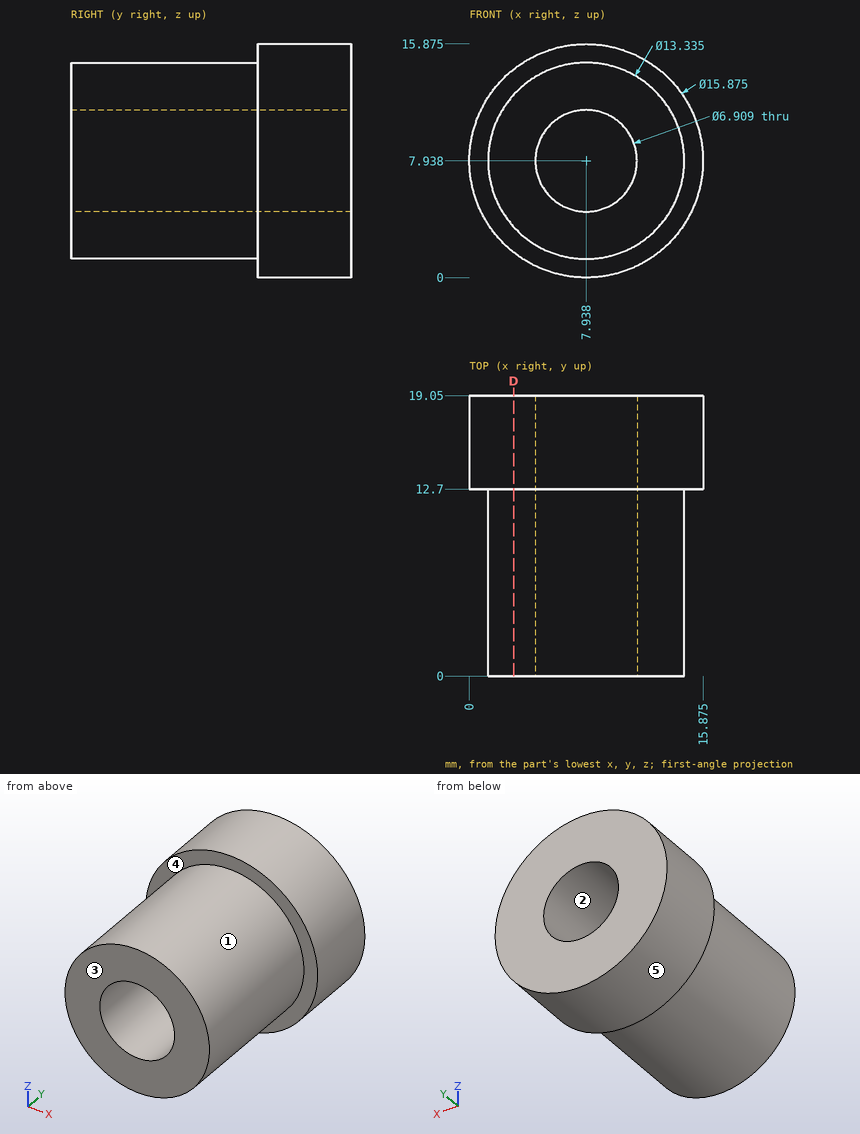
Design review of the part shown in the three views and the two pictorial views. Dimensions are in mm from the part's minimum x, y and z. A direction names the side the tool comes from. Give positions to 0.01 mm unless a question says otherwise; leave off trailing zeros. Write each loop counter-clockwise with the first axis right and the second up, starting at its lowest first coordinate (ties: lowest second). Pieces come first, ordered by that corner, then holes. Notation, with made-up numbers: M 76,33 L 103,33 A22 cw 103,48 Z; hole C 9,85 d4. An arc over 180 degrees is marked long. Answer in a Markdown table with one row per item.
Item 1: For P1, Ø3, axis at y = 15.5, z = 13, coming from the +X side; P2, Ø5, axis at x = 10.5, y = 10.5, coming from the -Z side; P3, Ø8, axis at x = 10.5, y = 10.5, coming from the -Z side; P4, Ø8, axis at y = 8, z = 11.5, coming from the +X side (1 decimal), all flat-tipped, find the tip position at first contact; note any pin that passes through.
Check sheet entries:
| item | result |
|---|---|
| P1 | x = 15.03 |
| P2 | z = 0.12 |
| P3 | z = 0 |
| P4 | x = 14.6 |
Item 2: Tool access review of the marked faces 4 and 5: name each direction out of +Z, -Z, +X, -X, +Y, -Y from which nothing blocks a thin tool from reaching the whole face with its end or side.
Check sheet entries:
| item | result |
|---|---|
| face 4 | -Y |
| face 5 | +Y, -Y |
Item 3: For line 1 along Z through (x, y) = (8, 8) (1 decimal); line 2 along Y through (x, z) = (4.25, 1.5), list the stretches that pass through material, from the lowest coordinate up.
Check sheet entries:
| item | result |
|---|---|
| line 1 | 1.3 to 4.5, 11.4 to 14.6 |
| line 2 | 12.7 to 19.05 |
Item 4: Draft analysis for pull direction X (two halves, no side actions). For the marked faces 1, 2 and 3, state which applies: +X half, -X half, draft (parallel to the pull), parting line (faces both ways), or undercut.
Check sheet entries:
| item | result |
|---|---|
| face 1 | parting line |
| face 2 | undercut |
| face 3 | draft |
Item 5: Add section D-D on x = 3. Give the boundary of the cut face in (y, z), plus the area to 3 significant figures.
Check sheet entries:
| item | result |
|---|---|
| outline | M 0,3.46 L 12.7,3.46 L 12.7,1.72 L 19.05,1.72 L 19.05,14.15 L 12.7,14.15 L 12.7,12.42 L 0,12.42 Z |
| area | 193 mm2 |
